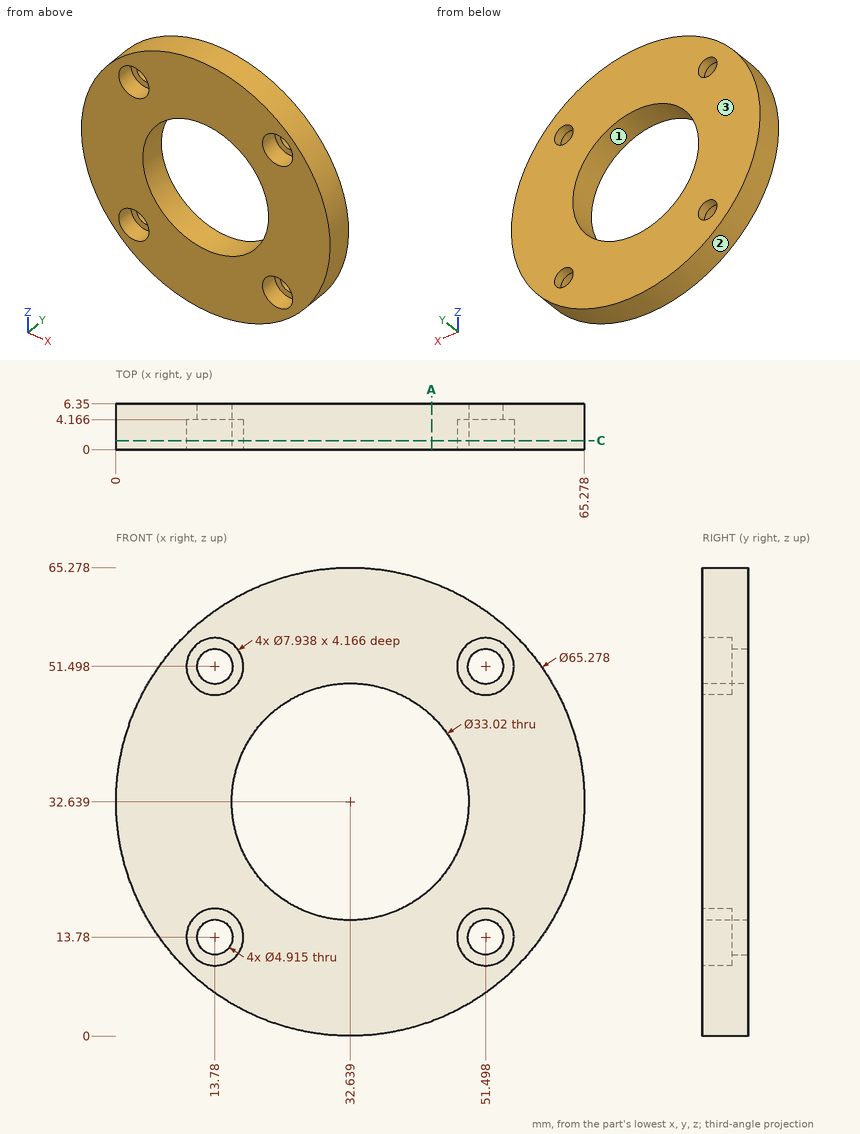
Geometry check sheet. Reference: drawing and pictorial views, mm from the part's lowest x, y, z. Round coordinates to 2 decimals unless told otherwise and drop trailing zeros. Loops run counter-clockwise (first coordinate to the right, second up) from the corner with the lowest first, then second, coordinate; pieces in that order, holes last. Notation, with made-up numbers: (12, 75.5) - (59, 75.5) arc R28 cw to (59, 95.5) - close; hole circle Ø1 at (-35.75, -18). An arc over 180 degrees is marked (long way). Use a Markdown table: item, result. Add a question column.
1. Section check C-C, the plane y = 1.25. Record the boundary of the cut face in (x, z), plus the area to 3 significant figures.
2. Thickness scan on probe 1 along Z at (x, y) = (14, 2.5) (1 decimal); probe 2 along Z at (x, y) = (33, 2) (1 decimal); probe 3 along Z at (x, y) = (12, 5.5) (1 decimal). Record the ranges inside material, lowest first. Write a range as [from, to].
3. Release check for a two-part mould opening along X. For the marked faces 1, 2 and 3 record: released by +X, released by -X, zero draft, split by the parting line, or undercut.
4. Gauge pin test, flat ends, axial feed: pin 1 (6.5 mm diameter, centred on x = 13.78, z = 13.78, fed in from -Y); pin 2 (1 mm diameter, centred on y = 4.5, z = 36.5, fed in from -X). Record the tip position at first contact, or that the pin passes through.
5. Section check A-A, the plane x = 44. Record the boundary of the cut face in (y, z).
Checks:
| question | item | result |
|---|---|---|
| 1 | outline | circle Ø65.28 at (32.64, 32.64); hole circle Ø7.94 at (13.78, 13.78); hole circle Ø7.94 at (13.78, 51.5); hole circle Ø33.02 at (32.64, 32.64); hole circle Ø7.94 at (51.5, 13.78); hole circle Ø7.94 at (51.5, 51.5) |
| 1 | area | 2,290 mm^2 |
| 2 | probe 1 | z = [5.8, 9.8], [17.7, 47.5], [55.5, 59.4] |
| 2 | probe 2 | z = [0, 16.1], [49.1, 65.3] |
| 2 | probe 3 | z = [7.4, 12.1], [15.5, 49.8], [53.2, 57.9] |
| 3 | face 1 | undercut |
| 3 | face 2 | split by the parting line |
| 3 | face 3 | zero draft |
| 4 | pin 1 | stops at y = 4.17 |
| 4 | pin 2 | stops at x = 0.17 |
| 5 | outline | (0, 2.04) - (6.35, 2.04) - (6.35, 20.66) - (0, 20.66) - close; (0, 44.62) - (6.35, 44.62) - (6.35, 63.24) - (0, 63.24) - close |
